from build123d import *

# Parameters (mm, degrees)
SKETCH_W      = 30
SKETCH_H      = 12
PAD_DEPTH     = 20
PAD001_DEPTH  = 10
SKETCH002_R   = 1.5
PAD002_DEPTH  = 5
CHAMFER_SIZE2 = 15
CHAMFER_SIZE  = 10
FILLET_R      = 3


with BuildPart() as part:
    # Sketch → Pad (new body)
    with BuildSketch(Plane.XY):
        with Locations((15, 6)):
            Rectangle(SKETCH_W, SKETCH_H)
    extrude(amount=PAD_DEPTH)

    # Sketch001 (on Face5 of Pad) → Pad001 (join)
    with BuildSketch(Plane(origin=(0, 0, 0), x_dir=(1, 0, 0), z_dir=(0, 0, -1))):
        Polygon((12, 0), (18, 0), (18, -3), (20, -3), (20, -8), (10, -8), (10, -3), (12, -3), align=None)
    extrude(amount=PAD001_DEPTH)

    # Sketch002 (on Face4 of Pad001) → Pad002 (join)
    with BuildSketch(Plane(origin=(0, 0, 0), x_dir=(1, 0, 0), z_dir=(0, 0, -1))):
        with Locations((3.5, -6)):
            Circle(SKETCH002_R)
        with Locations((26.5, -6)):
            Circle(SKETCH002_R)
    extrude(amount=PAD002_DEPTH)

    # Chamfer
    chamfer_edges = [part.edges().sort_by_distance(p)[0] for p in [
        (15, 12, 20),
    ]]
    chamfer_side = part.faces().sort_by_distance((15, 6, 20))[0]
    chamfer(chamfer_edges, length=CHAMFER_SIZE, length2=CHAMFER_SIZE2, reference=chamfer_side)

    # Fillet
    fillet_edges = [part.edges().sort_by_distance(p)[0] for p in [
        (0, 12, 2.5),
        (0, 0, 10),
        (30, 12, 2.5),
        (30, 0, 10),
    ]]
    fillet(fillet_edges, radius=FILLET_R)


solid = part.part
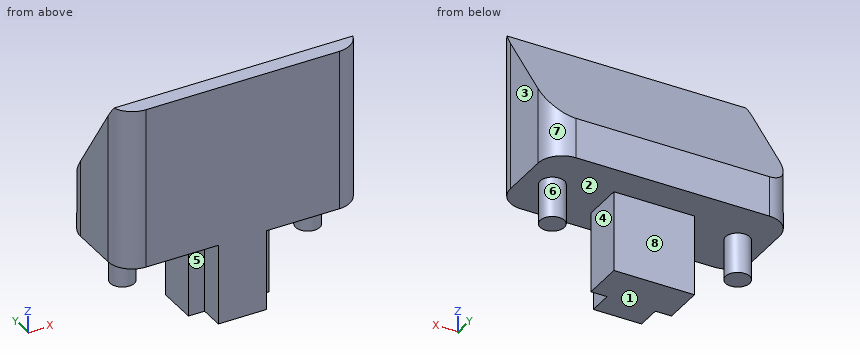
Source: CAD feature listing. Evaluate the final solid. Frame: model axes, mm. Face numbers are marked on the shaded views. A direction names the side the tool comes from. Coordinates: 2 decimals unless noted, no trailing zeros. Write each loop counter-clockwise with the first axis right and the second up, starting at its lowest first coordinate (ties: lowest second). Pieces come first, ordered by that corner, then holes. Notation, with made-up numbers: M 64.25,15.5 L 83.25,15.5 A17 cw 83.25,34.5 Z; hole C 79.25,39 d3. An arc over 180 degrees is marked long. Use a Markdown table: item, result.
1) Mould query, pull axis X, two halves, no side actions, for the marked faces 1, 2 and 3. Classes: pulls with the +X half, pulls with the -X half, needs draft (parallel to the pull), parting line crosses it, or undercut.
Conclusion:
| item | result |
|---|---|
| face 1 | needs draft |
| face 2 | undercut |
| face 3 | pulls with the +X half |
2) Ray query, L1, parallel to Y at x = 10.5, z = -1.25; L2, parallel to Z at x = 27.5, y = 1.5; L3, parallel to X at y = 3.25, z = -3.5. Return the intervals inside material, ascending.
Conclusion:
| item | result |
|---|---|
| L1 | y = 3 to 8 |
| L2 | z = 0 to 20 |
| L3 | x = 10 to 20 |
3) Section D-D, the plane x = 10.5. Output: boundary loops of the cut face in (y, z).
Conclusion:
| item | result |
|---|---|
| outline | M 0,0 L 3,0 L 3,-10 L 8,-10 L 8,0 L 12,0 L 12,5 L 2,20 L 0,20 Z |
4) First-contact query: pin 1 Ø1.5 at (y, z) = (2.5, -2.5) entering from -X; pin 2 Ø5.5 at (y, z) = (6.5, -7.5) entering from +X; pin 3 Ø1 at (x, z) = (11, -3.5) entering from -Y. Flat tips, straight axial feed; report the tip coordinate or a pass-through.
Conclusion:
| item | result |
|---|---|
| pin 1 | stops at x = 10 |
| pin 2 | stops at x = 28 |
| pin 3 | stops at y = 3 |
5) Reachability of the marked faces 4, 5, 6, 7 and 8 from +Z, -Z, +X, -X, +Y, -Y: full face, straight path, thin tool, end or side. Return the list, or none.
Conclusion:
| item | result |
|---|---|
| face 4 | -Z, +Y, -Y |
| face 5 | -Z, -X, -Y |
| face 6 | -Z |
| face 7 | +Z, -Z, +X, +Y |
| face 8 | -Z, +X, -X, +Y |
6) Section C-C, the plane y = 3.5. Output: boundary loops of the cut face in (x, z).
Conclusion:
| item | result |
|---|---|
| outline | M 0,0 L 10,0 L 10,-10 L 20,-10 L 20,0 L 30,0 L 30,17.75 L 0,17.75 Z |
7) Section B-B, the plane x = 21.5. Output: boundary loops of the cut face in (y, z).
Conclusion:
| item | result |
|---|---|
| outline | M 0,0 L 12,0 L 12,5 L 2,20 L 0,20 Z |
8) Section A-A, the plane z = -3. Output: boundary loops of the cut face in (x, y), then the cut area to 3 significant figures.
Conclusion:
| item | result |
|---|---|
| outline | C 3.5,6 d3; M 10,3 L 12,3 L 12,0 L 18,0 L 18,3 L 20,3 L 20,8 L 10,8 Z; C 26.5,6 d3 |
| area | 82.1 mm^2 |
